Work out the finished part from the listing and answer in its coordinate system (mm). A direction names the side the tool comes from. Round coordinates to 2 decimals unless told otherwise and drop trailing zeros. Order: outer loops, then holes, each group sorted by start corner. A loop starts at its lowest first (then second) coordinate and runs counter-clockwise, first axis right, second up. Notation, with made-up numbers: (19, 71.25) - (48, 71.25) arc R20 ccw to (48, 92.25) - close; hole circle Ø1 at (9, 25.5). An arc over 180 degrees is marked (long way). Put each result on its own line as item: value.
```python
from build123d import *

# Parameters (mm, degrees)
SKETCH1_W                  = 100
SKETCH1_H                  = 12.7
BOSS_EXTRUDE1_DEPTH        = 6.35
SKETCH2_W                  = 25.4
SKETCH2_H                  = 6.35
CUT_EXTRUDE1_DEPTH         = 13.7
F_6_32_TAPPED_HOLE1_D      = 2.7051
F_8_32_TAPPED_HOLE1_D      = 3.4544
F_8_32_TAPPED_HOLE1_DEPTH  = 10
F_8_32_TAPPED_HOLE1_TIP    = 1.037806461
F_2_0_221_DIAMETER_HOLE1_D = 2.54
F_2_56_TAPPED_HOLE2_D      = 1.778
F_2_56_TAPPED_HOLE2_DEPTH  = 5
F_2_56_TAPPED_HOLE2_TIP    = 0.53416509
FILLET2_R                  = 1


with BuildPart() as part:
    # Sketch1 → Boss-Extrude1 (new body, symmetric)
    with BuildSketch(Plane.XY):
        with Locations((50, 0)):
            Rectangle(SKETCH1_W, SKETCH1_H)
    extrude(amount=BOSS_EXTRUDE1_DEPTH, both=True)

    # Sketch2 → Cut-Extrude1 (cut, through all)
    with BuildSketch(Plane.XY.offset(6.35)):
        with Locations((12.7, 3.175)):
            Rectangle(SKETCH2_W, SKETCH2_H)
    extrude(amount=-CUT_EXTRUDE1_DEPTH, mode=Mode.SUBTRACT)

    # #6-32 Tapped Hole1 (through all)
    with Locations(Plane(origin=(0, 0, 0), x_dir=(-1, 0, 0), z_dir=(0, 1, 0))):
        with Locations((-17.7, 0), (-5, 0)):
            Hole(F_6_32_TAPPED_HOLE1_D / 2)

    # #8-32 Tapped Hole1
    with Locations(Plane(origin=(100, 0, 0), x_dir=(0, 0, -1), z_dir=(1, 0, 0))):
        with Locations((0, 0)):
            Hole(F_8_32_TAPPED_HOLE1_D / 2, depth=F_8_32_TAPPED_HOLE1_DEPTH)
            with Locations((0, 0, -(F_8_32_TAPPED_HOLE1_DEPTH + F_8_32_TAPPED_HOLE1_TIP / 2))):  # 118° drill point
                Cone(0, F_8_32_TAPPED_HOLE1_D / 2, F_8_32_TAPPED_HOLE1_TIP, mode=Mode.SUBTRACT)

    # #2 (0.221) Diameter Hole1 (through all)
    with Locations(Plane(origin=(0, 6.35, 0), x_dir=(-1, 0, 0), z_dir=(0, 1, 0))):
        with Locations((-35.4, -2.7686), (-76.675, -2.7686), (-76.675, 2.7686), (-35.4, 2.7686)):
            Hole(F_2_0_221_DIAMETER_HOLE1_D / 2)

    # #2-56 Tapped Hole2
    with Locations(Plane(origin=(0, 6.35, 0), x_dir=(-1, 0, 0), z_dir=(0, 1, 0))):
        with Locations((-84.76, 0), (-96.19, 0)):
            Hole(F_2_56_TAPPED_HOLE2_D / 2, depth=F_2_56_TAPPED_HOLE2_DEPTH)
            with Locations((0, 0, -(F_2_56_TAPPED_HOLE2_DEPTH + F_2_56_TAPPED_HOLE2_TIP / 2))):  # 118° drill point
                Cone(0, F_2_56_TAPPED_HOLE2_D / 2, F_2_56_TAPPED_HOLE2_TIP, mode=Mode.SUBTRACT)

    # Fillet2
    fillet2_edges = [part.edges().sort_by_distance(p)[0] for p in [
        (0, 0, 0),
    ]]
    fillet(fillet2_edges, radius=FILLET2_R)


solid = part.part
```
1) Straight lines are drawn through the part: L1, parallel to X at y = 1.75, z = -0.5; L2, parallel to Z at x = 17.7, y = -1.5; L3, parallel to X at y = 0.5, z = -3.25. For each, find the intervals that lie inside material, in ascending order. Write a range as from..to.
Findings below:
L1: x = 25.4..84.02, 85.5..95.45, 96.93..100
L2: z = -6.35..-1.35, 1.35..6.35
L3: x = 25.4..34.22, 36.58..75.5, 77.85..100
2) Given pin 1 Ø3.5 at (x, z) = (76.68, -2.77) entering from -Y; pin 2 Ø4 at (x, z) = (16, -1) entering from +Y; pin 3 Ø3 at (y, z) = (2.5, -3) entering from -X; pin 4 Ø1.1 at (x, z) = (84.76, 0) entering from +Y, each flat-ended and moving along its own axis, determine where each tip first touches the part or whether it passes through.
Findings below:
pin 1: stops at y = -6.35
pin 2: stops at y = 0
pin 3: stops at x = 25.4
pin 4: stops at y = 1.15
3) A cutting plane is placed at A-A on x = 5. Write down the section's boundary in (y, z).
Findings below:
outline: (-6.35, -6.35) - (0, -6.35) - (0, -1.35) - (-6.35, -1.35) - close; (-6.35, 1.35) - (0, 1.35) - (0, 6.35) - (-6.35, 6.35) - close
4) A cutting plane is placed at D-D on y = -4.25. Write down the section's boundary in (x, z) (3 decimals), then the cut area to 3 significant figures.
Findings below:
outline: (0, -6.35) - (100, -6.35) - (100, 6.35) - (0, 6.35) - close; hole circle Ø2.705 at (5, 0); hole circle Ø2.705 at (17.7, 0); hole circle Ø2.54 at (35.4, -2.769); hole circle Ø2.54 at (35.4, 2.769); hole circle Ø2.54 at (76.675, -2.769); hole circle Ø2.54 at (76.675, 2.769)
area: 1,240 mm2
5) A cutting plane is placed at B-B on y = 3. Write down the section's boundary in (x, z) (3 decimals).
Findings below:
outline: (25.4, -6.35) - (100, -6.35) - (100, 6.35) - (25.4, 6.35) - close; hole circle Ø2.54 at (35.4, -2.769); hole circle Ø2.54 at (35.4, 2.769); hole circle Ø2.54 at (76.675, -2.769); hole circle Ø2.54 at (76.675, 2.769); hole circle Ø1.778 at (84.76, 0); hole circle Ø1.778 at (96.19, 0)
6) A cutting plane is placed at C-C on x = 17.5. Write down the section's boundary in (y, z).
Findings below:
outline: (-6.35, -6.35) - (0, -6.35) - (0, -1.34) - (-6.35, -1.34) - close; (-6.35, 1.34) - (0, 1.34) - (0, 6.35) - (-6.35, 6.35) - close
7) For a pull along Y with two mould halves and no side action, classify faces 4 (the cylindrical face through (77.886, -0.089, -2.387)), 5 (the cylindrical face through (94.93, -1.686, -0.374)), 6 (the flat face through (62, 6.35, 0)) as pulls with the +Y half, pulls with the -Y half, needs draft (parallel to the pull), parting line crosses it, or undercut.
Findings below:
face 4: needs draft
face 5: undercut
face 6: pulls with the +Y half
8) For faces 1 (the flat face through (25.4, 3, 0)), 2 (the cylindrical face through (97.038, 3.881, 0.267)), 3 (the flat face through (49, 0, -6.35)), determine the directions among +Z, -Z, +X, -X, +Y, -Y from which every point of the face is accessible in a straight line to the end or side of a thin tool.
Findings below:
face 1: +Z, -Z, -X, +Y
face 2: +Y
face 3: -Z, +X, -X, +Y, -Y
